Autodesk Inventor part; units mm, degrees
ref_plane "YZ Plane" through (0, 0, 0) normal (1, 0, 0) x (0, 1, 0)
ref_plane "XZ Plane" through (0, 0, 0) normal (0, 1, 0) x (-1, 0, 0)
ref_plane "XY Plane" through (0, 0, 0) normal (0, 0, 1) x (1, 0, 0)
sketch "Sketch1" plane through (0, 0, 0) normal (0, 1, 0) x (-1, 0, 0)
  line L0 (0, 0) -> (228.6, 0)
  line L1 (228.6, 0) -> (228.6, -965.2)
  line L2 (228.6, -965.2) -> (0, -965.2)
  line L3 (0, -965.2) -> (0, 0)
  line L4 (0, -19.05) -> (209.55, -19.05)
  line L5 (209.55, -19.05) -> (209.55, -946.15)
  line L6 (209.55, -946.15) -> (0, -946.15)
  line L7 (0, -946.15) -> (0, -19.05)
  point P0 (0, -946.15)
  dimension "d0" = 228.6
  dimension "d1" = 965.2
  dimension "d2" = 19.05
  dimension "d3" = 19.05
  dimension "d4" = 19.05
extrude "Extrusion1" add sketch "Sketch1" along normal blind 457.2 contours L0 L1 L2 L3 L6 L5 L4
sketch "Sketch2" plane through (0, 0, 0) normal (0, -1, 0) x (1, 0, 0)
  line L0 (0, -19.05) -> (-209.55, -19.05)
  line L1 (-209.55, -19.05) -> (-209.55, -946.15)
  line L2 (-190.5, -19.05) -> (-209.55, -19.05)
  line L3 (-209.55, -19.05) -> (-209.55, -946.15)
  line L4 (-209.55, -946.15) -> (-190.5, -946.15)
  line L5 (-190.5, -946.15) -> (-190.5, -19.05)
  point P0 (0, 0)
  dimension "d7" = 19.05
extrude "Extrusion2" add sketch "Sketch2" against normal blind 76.2
sketch "Sketch3" plane through (-209.55, 457.2, -19.05) normal (1, 0, 0) x (0, 0, -1)
  line L0 (0, -381) -> (927.1, -381)
  line L1 (927.1, -381) -> (927.1, 0)
  line L2 (0, 0) -> (927.1, 0)
  line L3 (0, -381) -> (0, 0)
  line L4 (0, -457.2) -> (0, 0)
  line L5 (927.1, -457.2) -> (927.1, 0)
  line L6 (0, -101.6) -> (927.1, -101.6)
  line L7 (927.1, -101.6) -> (927.1, -120.65)
  line L8 (927.1, -120.65) -> (0, -120.65)
  line L9 (0, -120.65) -> (0, -101.6)
  point P0 (-19.05, -457.2)
  point P1 (0, -120.65)
  point P2 (927.1, -120.65)
  point P3 (927.1, -101.6)
  dimension "d10" = 19.05
  dimension "d11" = 101.6
extrude "Extrusion3" add sketch "Sketch3" along normal blind 203.2 contours L3 L6 L1 L8
sketch "Sketch4" plane through (-209.55, 336.55, -946.15) normal (0, -1, 0) x (1, 0, 0)
  line L0 (209.55, 927.1) -> (19.05, 927.1)
  line L1 (19.05, 0) -> (209.55, 0)
  line L2 (200.025, 927.1) -> (180.975, 927.1)
  line L3 (180.975, 927.1) -> (180.975, 0)
  line L4 (180.975, 0) -> (200.025, 0)
  line L5 (200.025, 0) -> (200.025, 927.1)
  line L6 (203.2, 927.1) -> (203.2, 0)
  point P0 (209.55, 946.15)
  point P1 (200.025, 0)
  dimension "d14" = 19.05
  dimension "d15" = 3.175
extrude "Extrusion4" add sketch "Sketch4" along normal blind 38.1 contours L5 L1 L3 L0
fillet "Fillet1" radius 3.175 4 edges at (-6.35, 355.6, -482.6) (-6.35, 336.55, -482.6) (0, 457.2, -9.525) (0, 457.2, -955.675)
properties part number "Shelf" material "Wood (Birch)"
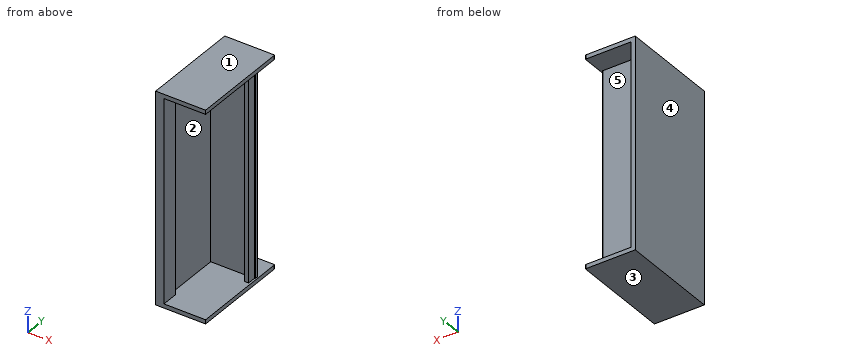
The listing builds one solid part. Answer for the finished solid, in the listing's coordinates (mm). Face numbers are marked on the shaded views. A direction names the side the tool comes from. Coordinates: 2 decimals unless noted, no trailing zeros. Write each loop counter-clockwise with the first axis right and the second up, starting at its lowest first coordinate (ties: lowest second). Pieces come first, ordered by that corner, then holes. Notation, with made-up numbers: M -39,35.5 L -11,35.5 A16 ccw -11,47.5 Z; hole C 47.25,12.5 d7. An arc over 180 degrees is marked long. Use a Markdown table: item, result. Add a question column.
1. Straight lines are drawn through the part: line 1 along Z through (x, y) = (-137, 415.5); line 2 along X through (y, z) = (307.5, -700.5) (3 decimals); line 3 along X through (y, z) = (126, -644.5). For each, find the intervals that lie inside material, in ascending order. Write a range as [from, to].
2. Section A-A (x = -71) is taken. Give the vertices of the cut face in (y, z), plus the area to 3 significant figures.
3. Section B-B (y = 387.5) is taken. Give the vertices of the cut face in (x, z).
4. For a pull along Z with two mould halves and no side action, classify the marked faces 1, 2 and 3 as +Z half, -Z half, draft (parallel to the pull), parting line (faces both ways), or undercut.
5. Which of the six approach directions +Z, -Z, +X, -X, +Y, -Y give full straight-line access (tool end or side, diameter ignored) to the marked faces 4 and 5?
6. Given P1, Ø4, axis at x = -67, y = 405, coming from the +Z side; P2, Ø23, axis at y = 22, z = -341.5, coming from the +X side; P3, Ø1.5, axis at x = -98, z = -757, coming from the -Y side; P4, Ø4, axis at y = 359.5, z = -545.5, coming from the +X side, each flat-ended and moving along its own axis, determine where each tip first touches the part or whether it passes through.
Data:
| question | item | result |
|---|---|---|
| 1 | line 1 | z = [-965.2, -946.15], [-19.05, 0] |
| 1 | line 2 | x = [-228.6, -209.55], [-28.575, -9.525] |
| 1 | line 3 | x = [-228.6, -209.55] |
| 2 | outline | M 0,-965.2 L 457.2,-965.2 L 457.2,-946.15 L 355.6,-946.15 L 355.6,-19.05 L 457.2,-19.05 L 457.2,0 L 0,0 L 0,-19.05 L 336.55,-19.05 L 336.55,-946.15 L 0,-946.15 Z |
| 2 | area | 35,100 mm2 |
| 3 | outline | M -228.6,-965.2 L 0,-965.2 L 0,-946.15 L -209.55,-946.15 L -209.55,-19.05 L 0,-19.05 L 0,0 L -228.6,0 Z |
| 4 | face 1 | +Z half |
| 4 | face 2 | undercut |
| 4 | face 3 | -Z half |
| 5 | face 4 | +Z, -Z, -X, +Y, -Y |
| 5 | face 5 | +X, +Y |
| 6 | P1 | stops at z = 0 |
| 6 | P2 | stops at x = -190.5 |
| 6 | P3 | stops at y = 336.55 |
| 6 | P4 | stops at x = -209.55 |
